The drawing under review shows one solid part. Ordinate dimensions are in mm from its lowest x, y, z. A direction names the side the tool comes from. Give positions to 0.01 mm unless a question says otherwise; leave off trailing zeros. Write each loop counter-clockwise with the first axis right and the second up, starting at its lowest first coordinate (ties: lowest second). Pieces come first, ordered by that corner, then holes.
Q1. Insertion check: P1, Ø6, axis at x = 9, y = 5.5, coming from the -Z side; P2, Ø1, axis at x = 6.5, z = 3.5, coming from the +Y side. Each pin has a flat end and moves straight along its axis. Give the tip position at first contact, or say it passes through.
Q2. We need section B-B (z = 3.5). Write out the cut boundary in (x, y) (1 decimal), then the cut area to 3 significant figures.
Q3. We need section A-A (z = 1.3). Write out the cut boundary in (x, y) (1 decimal), then the cut area to 3 significant figures.
Q4. Machinability: for the marked faces 1 and 2, which of the approach directions +Z, -Z, +X, -X, +Y, -Y give a long, thin tool a straight path to every point of the face, cutting with its end or side? Answer none if there is none.
Q5. For line 1 (Z direction, x = 13.25, y = 3); line 2 (X direction, y = 13.25, z = 2.2); line 3 (Y direction, x = 12.25, z = 1.15), list the stretches that pass through material, from the lowest coordinate up.
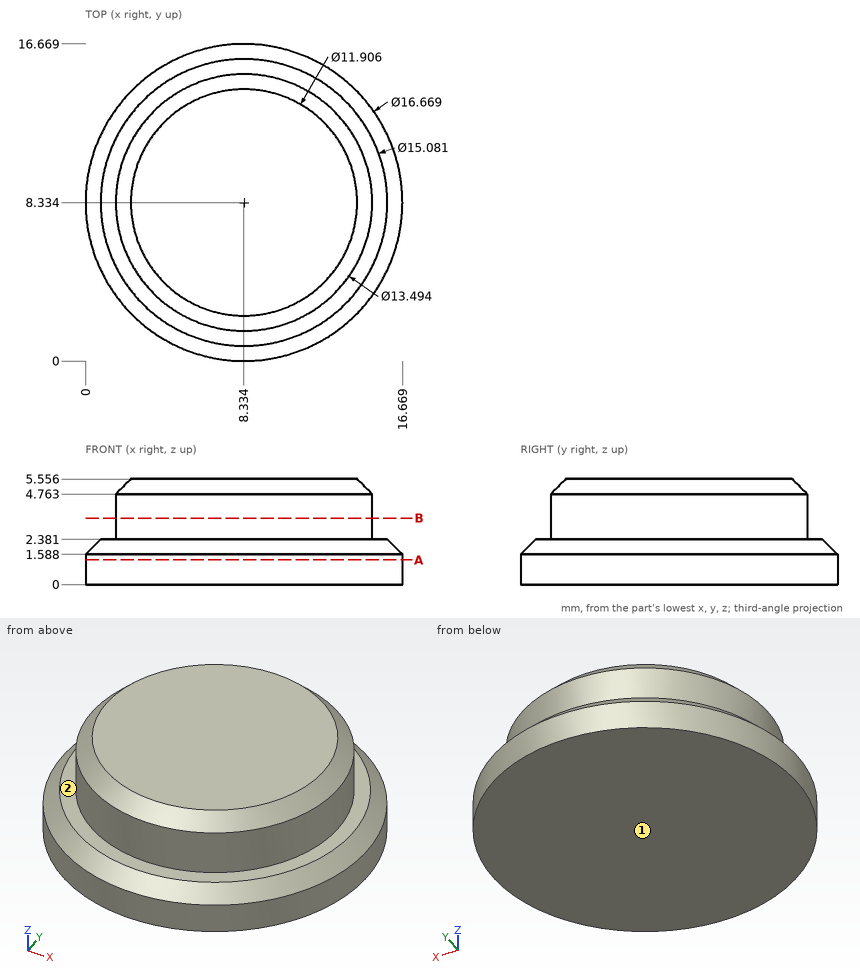
Computed:
1. P1: stops at z = 0
1. P2: stops at y = 14.95
2. outline: circle Ø13.5 at (8.3, 8.3)
2. area: 143 mm2
3. outline: circle Ø16.7 at (8.3, 8.3)
3. area: 218 mm2
4. face 1: -Z, +X, -X, +Y, -Y
4. face 2: +Z
5. line 1: z = 0 to 2.38
5. line 2: x = 2.38 to 14.29
5. line 3: y = 0.98 to 15.69
